Geometry check sheet. Reference: the model listing, model coordinates, mm. A direction names the side the tool comes from. Round coordinates to 2 decimals unless told otherwise and drop trailing zeros. Order: outer loops, then holes, each group sorted by start corner. A loop starts at its lowest first (then second) coordinate and runs counter-clockwise, first axis right, second up. Notation, with made-up numbers: (20.25, 86) - (78.25, 86) arc R21 ccw to (78.25, 113) - close; hole circle Ø10 at (-28, -22.75). An arc over 180 degrees is marked (long way). Write each question's results on one line, items separated by ' | '.
```python
from build123d import *

# Parameters (mm, degrees)
SKIZZE1_R                       = 12.5
AUFSATZ_LINEAR_AUSTRAGEN1_DEPTH = 4
DURCHGANGSLOCH_F_R_M31_D        = 3.4
SCHNITT_LINEAR_AUSTRAGEN1_DEPTH = 5
SCHNITT_LINEAR_AUSTRAGEN2_DEPTH = 5


with BuildPart() as part:
    # Skizze1 → Aufsatz-Linear austragen1 (new body)
    with BuildSketch(Plane.XY):
        with BuildLine():
            Line((60.618791136, -25.122399911), (53.121982765, -24.466514166))
            ThreePointArc((53.121982765, -24.466514166), (52.087524265, -24.556394327), (51.145668645, -24.99353369))
            ThreePointArc((51.145668645, -24.99353369), (47.84965812, -26.988212977), (44.325198534, -28.544045699))
            ThreePointArc((44.325198534, -28.544045699), (43.426888741, -29.064835818), (42.759922204, -29.860661471))
            Line((42.759922204, -29.860661471), (38.997199723, -36.377887981))
            Line((38.997199723, -36.377887981), (28.997199723, -36.377887981))
            Line((28.997199723, -36.377887981), (26.399123512, -31.877887981))
            ThreePointArc((26.399123512, -31.877887981), (25.301047301, -30.77981177), (23.801047301, -30.377887981))
            Line((23.801047301, -30.377887981), (-36.002800277, -30.377887981))
            ThreePointArc((-36.002800277, -30.377887981), (-66.002800277, -0.377887981), (-36.002800277, 29.622112019))
            Line((-36.002800277, 29.622112019), (23.801047301, 29.622112019))
            ThreePointArc((23.801047301, 29.622112019), (25.301047301, 30.024035807), (26.399123512, 31.122112019))
            Line((26.399123512, 31.122112019), (28.997199723, 35.622112019))
            Line((28.997199723, 35.622112019), (38.997199723, 35.622112019))
            Line((38.997199723, 35.622112019), (42.759922204, 29.104885508))
            ThreePointArc((42.759922204, 29.104885508), (43.426888741, 28.309059855), (44.325198534, 27.788269736))
            ThreePointArc((44.325198534, 27.788269736), (47.84965812, 26.232437014), (51.145668645, 24.237757727))
            ThreePointArc((51.145668645, 24.237757727), (52.087524265, 23.800618365), (53.121982765, 23.710738204))
            Line((53.121982765, 23.710738204), (60.618791136, 24.366623949))
            Line((60.618791136, 24.366623949), (66.3545555, 16.175103506))
            Line((66.3545555, 16.175103506), (63.173776116, 9.353900106))
            ThreePointArc((63.173776116, 9.353900106), (62.906383033, 8.372251699), (62.982460357, 7.357685339))
            ThreePointArc((62.982460357, 7.357685339), (62.618871056, 5.641491574), (61.042300943, 4.872112019))
            Line((61.042300943, 4.872112019), (47.785287356, 4.872112019))
            Line((47.785287356, 4.872112019), (39.265024534, 7.815111963))
            ThreePointArc((39.265024534, 7.815111963), (18.497199723, -0.377887981), (39.265024534, -8.570887926))
            Line((39.265024534, -8.570887926), (47.785287356, -5.627887981))
            Line((47.785287356, -5.627887981), (61.042300943, -5.627887981))
            ThreePointArc((61.042300943, -5.627887981), (62.618871056, -6.397267536), (62.982460357, -8.113461302))
            ThreePointArc((62.982460357, -8.113461302), (62.906383033, -9.128027661), (63.173776116, -10.109676068))
            Line((63.173776116, -10.109676068), (66.3545555, -16.930879469))
            Line((66.3545555, -16.930879469), (60.618791136, -25.122399911))
        make_face()
        with Locations((-36.002800277, -0.377887981)):
            Circle(SKIZZE1_R, mode=Mode.SUBTRACT)
    extrude(amount=AUFSATZ_LINEAR_AUSTRAGEN1_DEPTH)

    # Durchgangsloch für M31 (through all)
    with Locations(Plane.XY.offset(4)):
        with Locations((33.997199723, 32.622112019), (61.029217185, 18.550134418), (61.029217185, -19.305910381), (33.997199723, -33.377887981)):
            Hole(DURCHGANGSLOCH_F_R_M31_D / 2)

    # Skizze6 → Schnitt-Linear austragen1 (cut, through all)
    with BuildSketch(Plane.XY.offset(4)):
        with BuildLine():
            ThreePointArc((-30.28289938, 20.96907278), (-34.557391121, 21.674794222), (-38.887429125, 21.533043455))
            ThreePointArc((-38.887429125, 21.533043455), (-40.69535833, 19.176904242), (-38.339219117, 17.368975037))
            ThreePointArc((-38.339219117, 17.368975037), (-34.832084263, 17.483786745), (-31.369939369, 16.912184309))
            ThreePointArc((-31.369939369, 16.912184309), (-28.797975139, 18.39710855), (-30.28289938, 20.96907278))
        make_face()
        with BuildLine():
            ThreePointArc((-14.655839516, 5.342012915), (-16.181912689, 9.396692073), (-18.469691456, 13.0757396))
            ThreePointArc((-18.469691456, 13.0757396), (-21.414132472, 13.463382613), (-21.801775485, 10.518941598))
            ThreePointArc((-21.801775485, 10.518941598), (-19.948778203, 7.539079574), (-18.712727986, 4.254972926))
            ThreePointArc((-18.712727986, 4.254972926), (-16.140763756, 2.770048686), (-14.655839516, 5.342012915))
        make_face()
        with BuildLine():
            ThreePointArc((-20.375740412, -16.004947846), (-17.627321845, -12.655990131), (-15.585062608, -8.835191837))
            ThreePointArc((-15.585062608, -8.835191837), (-16.721574418, -6.09140961), (-19.465356645, -7.227921421))
            ThreePointArc((-19.465356645, -7.227921421), (-21.119494216, -10.322595152), (-23.345588893, -13.035099365))
            ThreePointArc((-23.345588893, -13.035099365), (-23.345588893, -16.004947846), (-20.375740412, -16.004947846))
        make_face()
        with BuildLine():
            ThreePointArc((-41.722701173, -21.724848742), (-37.448209433, -22.430570185), (-33.118171429, -22.288819418))
            ThreePointArc((-33.118171429, -22.288819418), (-31.310242223, -19.932680205), (-33.666381436, -18.124751))
            ThreePointArc((-33.666381436, -18.124751), (-37.17351629, -18.239562707), (-40.635661184, -17.667960272))
            ThreePointArc((-40.635661184, -17.667960272), (-43.207625414, -19.152884512), (-41.722701173, -21.724848742))
        make_face()
        with BuildLine():
            ThreePointArc((-57.349761038, -6.097788878), (-55.823687864, -10.152468035), (-53.535909097, -13.831515562))
            ThreePointArc((-53.535909097, -13.831515562), (-50.591468081, -14.219158576), (-50.203825068, -11.274717561))
            ThreePointArc((-50.203825068, -11.274717561), (-52.05682235, -8.294855536), (-53.292872567, -5.010748889))
            ThreePointArc((-53.292872567, -5.010748889), (-55.864836797, -3.525824648), (-57.349761038, -6.097788878))
        make_face()
        with BuildLine():
            ThreePointArc((-51.629860141, 15.249171883), (-54.378278708, 11.900214168), (-56.420537945, 8.079415874))
            ThreePointArc((-56.420537945, 8.079415874), (-55.284026135, 5.335633648), (-52.540243909, 6.472145458))
            ThreePointArc((-52.540243909, 6.472145458), (-50.886106337, 9.56681919), (-48.66001166, 12.279323402))
            ThreePointArc((-48.66001166, 12.279323402), (-48.66001166, 15.249171883), (-51.629860141, 15.249171883))
        make_face()
    extrude(amount=-SCHNITT_LINEAR_AUSTRAGEN1_DEPTH, mode=Mode.SUBTRACT)

    # Skizze7 → Schnitt-Linear austragen2 (cut, through all)
    with BuildSketch(Plane.XY.offset(4)):
        with BuildLine():
            Line((16.940850537, 17.278461205), (22.940850537, 17.278461205))
            ThreePointArc((22.940850537, 17.278461205), (25.040850537, 15.178461205), (22.940850537, 13.078461205))
            Line((22.940850537, 13.078461205), (16.940850537, 13.078461205))
            ThreePointArc((16.940850537, 13.078461205), (14.840850537, 15.178461205), (16.940850537, 17.278461205))
        make_face()
        with BuildLine():
            Line((48.05354891, 17.278461205), (54.05354891, 17.278461205))
            ThreePointArc((54.05354891, 17.278461205), (56.15354891, 15.178461205), (54.05354891, 13.078461205))
            Line((54.05354891, 13.078461205), (48.05354891, 13.078461205))
            ThreePointArc((48.05354891, 13.078461205), (45.95354891, 15.178461205), (48.05354891, 17.278461205))
        make_face()
        with BuildLine():
            Line((54.05354891, -17.984237167), (48.05354891, -17.984237167))
            ThreePointArc((48.05354891, -17.984237167), (46.00354891, -15.934237167), (48.05354891, -13.884237167))
            Line((48.05354891, -13.884237167), (54.05354891, -13.884237167))
            ThreePointArc((54.05354891, -13.884237167), (56.10354891, -15.934237167), (54.05354891, -17.984237167))
        make_face()
        with BuildLine():
            Line((22.940850537, -18.034237167), (16.940850537, -18.034237167))
            ThreePointArc((16.940850537, -18.034237167), (14.840850537, -15.934237167), (16.940850537, -13.834237167))
            Line((16.940850537, -13.834237167), (22.940850537, -13.834237167))
            ThreePointArc((22.940850537, -13.834237167), (25.040850537, -15.934237167), (22.940850537, -18.034237167))
        make_face()
    extrude(amount=-SCHNITT_LINEAR_AUSTRAGEN2_DEPTH, mode=Mode.SUBTRACT)


solid = part.part
```
(1) Draft check along X on faces 6 (the face through (-65.996, -1.038, 1.972)), 7 (the face through (40.85, 32.41, 1.97)), 8 (the face through (51, 13.078, 2)), 9 (the face through (-7, 29.622, 2)). Enter one of: released by +X, released by -X, zero draft, split by the parting line, or undercut.
Answers follow:
face 6: released by -X | face 7: released by +X | face 8: undercut | face 9: zero draft
(2) Depth check by flat-ended pin: pin 1 Ø1.2 at (x, z) = (7, 2) entering from -Y; pin 2 Ø1 at (x, z) = (45.5, 3) entering from -Y; pin 3 Ø1.2 at (x, z) = (4, 1.5) entering from +Y. Enter the tip coordinate at first touch or a pass-through.
Answers follow:
pin 1: y = -30.38 | pin 2: y = -28.29 | pin 3: y = 29.62
(3) Section check C-C (z = 2.2). Give the number of separate pieces and of enclosed holes in the cut face, then the cut area to 3 significant figures.
Answers follow:
separate pieces: 1 | enclosed holes: 15 | area: 5,710 mm²
(4) Material ranges on line 1 (X direction, y = -5.5, z = 3.6); line 2 (X direction, y = 3.5, z = 1.3); line 3 (X direction, y = -11.5, z = 0.45), recorded low to high.
Answers follow:
line 1: -65.56 to -57.42, -53.15 to -47.41, -24.6 to 19.65 | line 2: -65.75 to -47.89, -24.12 to -18.33, -15.03 to 19.14 | line 3: -63.86 to -55.1, -50.05 to -41.71, -30.3 to -21.98, -16.91 to 25.99, 35 to 63.82
(5) Section check B-B (x = 0). Record the cut outline in (y, z).
Answers follow:
outline: (-30.38, 0) - (29.62, 0) - (29.62, 4) - (-30.38, 4) - close
(6) Section check A-A (y = -2). Record the cut outline in (x, z), then the cut area to 3 significant figures.
Answers follow:
outline: (-65.96, 0) - (-48.4, 0) - (-48.4, 4) - (-65.96, 4) - close; (-23.61, 0) - (18.61, 0) - (18.61, 4) - (-23.61, 4) - close | area: 239 mm²
(7) Access from +Z, -Z, +X, -X, +Y, -Y to the whole of each face (thin tool, end or side, straight path). Record for faces 1 (the face through (56.92, -24.8, 1.97)), 2 (the face through (64.74, -13.47, 1.97)), 3 (the face through (20, -18.034, 2)), 4 (the face through (-6, -30.378, 2)), 5 (the face through (34, 35.622, 2)).
Answers follow:
face 1: +Z, -Z, -Y | face 2: +Z, -Z, +X | face 3: +Z, -Z | face 4: +Z, -Z, -X, -Y | face 5: +Z, -Z, +X, -X, +Y
